Model file for the job. Use its own axes, mm. Give positions to 0.01 mm unless a question says otherwise; leave off trailing zeros. Order: outer loops, then holes, each group sorted by start corner. A loop starts at its lowest first (then second) coordinate and runs counter-clockwise, first axis right, second up. Notation, with made-up numbers: M 4.5,79.25 L 34.5,79.25 A32 cw 34.5,106.25 Z; hole C 87.5,32 d8. An arc over 180 degrees is marked long. Return JSON: item names as keys, results as strings. Group by question number.
1. Slice it at A-A on y = 0. List the corners of the cut face in (x, z), then the cut area to 3 significant figures.
2. Pin check, flat tips, straight feed: pin 1 (1 mm diameter, centred on x = -31.5, y = -18.5, fed in from -Z); pin 2 (1.5 mm diameter, centred on y = -24, z = 4.5, fed in from +X); pin 3 (1.5 mm diameter, centred on x = -24, z = 0.5, fed in from -Y). Stop position of each tip, or through.
3. Slice it at B-B on z = 3.95. List the corners of the cut face in (x, y), then the cut area to 3 significant figures.
4. Wall check: probe 1 along Y at (x, z) = (-19.5, 3.8); probe 2 along Y at (x, z) = (0, 3.65); probe 3 along Z at (x, y) = (-39.5, 8). Give the ranges that are in metal, low to high. Write a range as [from, to].
from build123d import *

# Parameters (mm, degrees)
F0_R     = 46
F0_R_2   = 42
F0_R_3   = 38
F1_DEPTH = 3
F2_DEPTH = 6
F4_SIZE  = 1


# Not quite as in the source:
# - a fillet or chamfer that OpenCascade refuses, or shapes differently, is made with other operations: its cross-section is extruded or revolved along the edge and cut away or added


with BuildPart() as f1:
    # F0 (on Top) → F1 (new body)
    with BuildSketch(Plane.XY):
        Circle(F0_R)
        Circle(F0_R_2, mode=Mode.SUBTRACT)
        Circle(F0_R_2)
        Circle(F0_R_3, mode=Mode.SUBTRACT)
        Circle(F0_R_3)
    extrude(amount=F1_DEPTH)

    # F0 (on Top) → F2 (join)
    with BuildSketch(Plane.XY):
        Circle(F0_R)
        Circle(F0_R_2, mode=Mode.SUBTRACT)
        Circle(F0_R_3)
    extrude(amount=F2_DEPTH)

    # F3: fillet of radius 5 on 1 edges, made by hand

    # F3_s1 → F3_t2 (revolve, cut)
    with BuildSketch(Plane.XZ):
        with BuildLine():
            ThreePointArc((46, 1.1010205144), (44.8729833462, 4.2632981746), (42, 6))
            Line((42, 6), (46, 6))
            Line((46, 6), (46, 1.1010205144))
        make_face()
    revolve(axis=Axis((0, 0, 6), (0, 0, 1)), mode=Mode.SUBTRACT)

    # F4
    f4_edges = [f1.edges().sort_by_distance(p)[0] for p in [
        (-38, 0, 6),
    ]]
    chamfer(f4_edges, length=F4_SIZE)


solid = f1.part
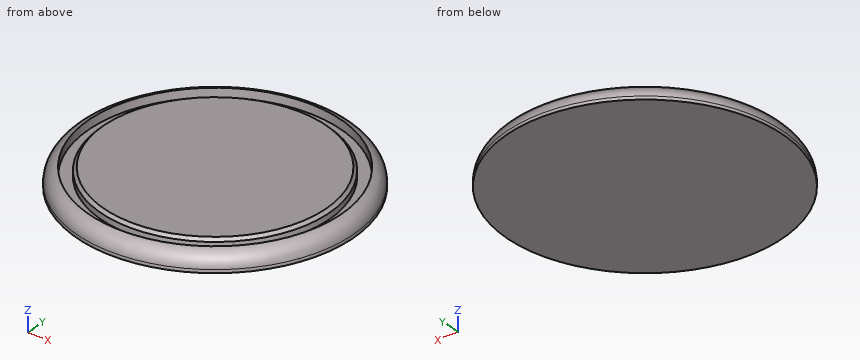
Result:
{
 "1": {"outline": "M -46,0 L 46,0 L 46,1.1 A5 ccw 42,6 L 42,3 L 38,3 L 38,5 L 37,6 L -37,6 L -38,5 L -38,3 L -42,3 L -42,6 A5 ccw -46,1.1 Z", "area": "517 mm2"},
 "2": {"pin 1": "stops at z = 0", "pin 2": "stops at x = 38.51", "pin 3": "stops at y = -39.69"},
 "3": {"outline": "C 0,0 d90.22; C 0,0 d76; hole C 0,0 d84", "area": "5,390 mm2"},
 "4": {"probe 1": "y = [-40.79, -37.2], [-32.62, 32.62], [37.2, 40.79]", "probe 2": "y = [-45.3, -42], [-38, 38], [42, 45.3]", "probe 3": "z = [0, 3]"}
}
